CAD build for the part. Positions are in the model's coordinates, mm. A direction names the side the tool comes from. Round coordinates to 2 decimals unless told otherwise and drop trailing zeros. Loops run counter-clockwise (first coordinate to the right, second up) from the corner with the lowest first, then second, coordinate; pieces in that order, holes last. Notation, with made-up numbers: M -25.5,16.5 L 31.5,16.5 A11 cw 31.5,33.5 Z; hole C 44,66.5 d10. An arc over 180 degrees is marked long. Use a Markdown table: item, result. Add a question column.
(1) Which spindle directions (+Z, -Z, +X, -X, +Y, -Y) get a long thin tool onto all of the face, cutting with end or side? Do faces 1 (the face through (-2, 5, 5)), 2 (the face through (-2.17, -9.76, -0.99)). Say none if no direction does.
(2) Band-saw the part on C-C, the plane z = 7.25. Write the cut outline in (x, y).
(3) Flat gauge pins, fed straight in: P1, Ø1.5, axis at x = 7.5, y = 5.5, coming from the +Z side; P2, Ø2, axis at x = -5, z = 1.5, coming from the +Y side; P3, Ø7, axis at x = -1, y = -1.5, coming from the +Z side. Where does each tip first touch, or does it go through?
(4) Band-saw the part on A-A, the plane y = 0. Write the cut outline in (x, z), and give its area (3 significant figures).
(5) Wall check: L1, parallel to Y at x = 0, z = 8.95; L2, parallel to Y at x = 0, z = -0.75; L3, parallel to Z at x = -4, y = -5.25. Give the ranges that are in metal, low to high.
(6) Band-saw the part on B-B, the plane z = 3.5. Write the cut outline in (x, y) (3 decimals).
(7) Two-plate mould, pull along Y, no slides. Class faces 3 (the face through (4.919, 7.715, 4.437)), 4 (the face through (4.893, 0, 3)), 5 (the face through (3, -7, 10)), 6 (the face through (-2.41, 4.26, 2.54)): released by +Y, released by -Y, zero draft, split by the parting line, or undercut.
from build123d import *

# Parameters (mm, degrees)
F0_R     = 10
F1_DEPTH = 2
F2_R     = 9.15
F3_DEPTH = 5
F5_DEPTH = 5
F6_R     = 9.15
F6_R_2   = 7.15
F7_DEPTH = 5
F8_R     = 3.1
F9_DEPTH = 12.001
F10_R    = 1


with BuildPart() as f1:
    # F0 (on Top) → F1 (new body)
    with BuildSketch(Plane.XY):
        Circle(F0_R)
    extrude(amount=-F1_DEPTH)

    # F2 (on face) → F3 (join)
    with BuildSketch(Plane.XY):
        Circle(F2_R)
    extrude(amount=F3_DEPTH)

    # F4 (on face) → F5 (cut)
    with BuildSketch(Plane.XY.offset(5)):
        Polygon((4.893044, 2.825), (0, 5.65), (-4.893044, 2.825), (-4.893044, -2.825), (0, -5.65), (4.893044, -2.825), align=None)
    extrude(amount=-F5_DEPTH, mode=Mode.SUBTRACT)

    # F6 (on face) → F7 (join)
    with BuildSketch(Plane.XY.offset(5)):
        Circle(F6_R)
        Circle(F6_R_2, mode=Mode.SUBTRACT)
    extrude(amount=F7_DEPTH)

    # F8 (on face) → F9 (cut, through all)
    with BuildSketch(Plane(origin=(0, 0, -2), x_dir=(1, 0, 0), z_dir=(0, 0, -1))):
        Circle(F8_R)
    extrude(amount=-F9_DEPTH, mode=Mode.SUBTRACT)

    # F10
    f10_edges = [f1.edges().sort_by_distance(p)[0] for p in [
        (-9.15, 0, 10),
    ]]
    fillet(f10_edges, radius=F10_R)


solid = f1.part
Return value:
| question | item | result |
|---|---|---|
| 1 | face 1 | +Z |
| 1 | face 2 | +Z, -Z |
| 2 | outline | C 0,0 d18.3; hole C 0,0 d14.3 |
| 3 | P1 | z = 9.92 |
| 3 | P2 | y = 8.23 |
| 3 | P3 | z = 5 |
| 4 | outline | M -10,-2 L -3.1,-2 L -3.1,0 L -4.89,0 L -4.89,5 L -7.15,5 L -7.15,10 L -8.15,10 A1 ccw -9.15,9 L -9.15,0 L -10,0 Z; M 3.1,-2 L 10,-2 L 10,0 L 9.15,0 L 9.15,9 A1 ccw 8.15,10 L 7.15,10 L 7.15,5 L 4.89,5 L 4.89,0 L 3.1,0 Z |
| 4 | area | 89.7 mm^2 |
| 5 | L1 | -9.15 to -7.15, 7.15 to 9.15 |
| 5 | L2 | -10 to -3.1, 3.1 to 10 |
| 5 | L3 | -2 to 5 |
| 6 | outline | C 0,0 d18.3; hole M -4.893,-2.825 L 0,-5.65 L 4.893,-2.825 L 4.893,2.825 L 0,5.65 L -4.893,2.825 Z |
| 7 | face 3 | split by the parting line |
| 7 | face 4 | undercut |
| 7 | face 5 | zero draft |
| 7 | face 6 | undercut |
